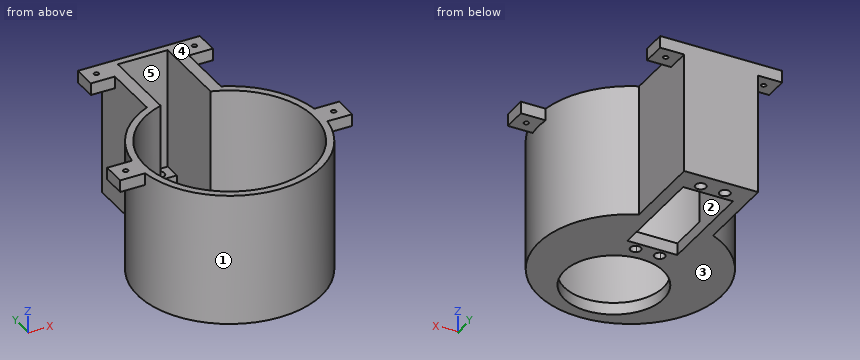
Autodesk Inventor part; units mm, degrees
ref_plane "YZ Plane" through (0, 0, 0) normal (1, 0, 0) x (0, 1, 0)
ref_plane "XZ Plane" through (0, 0, 0) normal (0, 1, 0) x (-1, 0, 0)
ref_plane "XY Plane" through (0, 0, 0) normal (0, 0, 1) x (1, 0, 0)
ref_plane "Work Plane1" through (0, 0, 0) normal (0, 0, 1) x (1, 0, 0)
sketch "Sketch1" plane through (0, 0, 0) normal (0, 0, 1) x (1, 0, 0)
  line L0 (10.3879, -20.2759) -> (10.3879, 20.2759)
  line L1 (-9.35, -21.3138) -> (9.35, -21.3138)
  line L2 (-10.3879, -21.3138) -> (10.3879, -21.3138)
  line L3 (10.3879, -21.3138) -> (10.3879, 21.3138)
  line L4 (10.3879, 21.3138) -> (-10.3879, 21.3138)
  line L5 (-10.3879, 21.3138) -> (-10.3879, -21.3138)
  line L6 (-10.3879, -21.3138) -> (10.3879, 21.3138) construction
  line L7 (10.3879, -21.3138) -> (-10.3879, 21.3138) construction
  line L8 (-15.3879, 31.3138) -> (15.3879, 31.3138)
  arc A0 (-6.25, 26.7) -> (-3.75, 26.7) centre (-5, 24.8896) ccw
  arc A1 (3.75, 26.7) -> (6.25, 26.7) centre (5, 24.8896) ccw
  arc A2 (-3.75, -26.7) -> (-6.25, -26.7) centre (-5, -24.8896) ccw
  arc A3 (6.25, -26.7) -> (3.75, -26.7) centre (5, -24.8896) ccw
  circle A4 centre (-5, 24.8896) radius 2.2
  circle A5 centre (5, 24.8896) radius 2.2
  circle A6 centre (-5, -24.8896) radius 2.2
  circle A7 centre (5, -24.8896) radius 2.2
  circle A8 centre (0, -50.7404) radius 20.6245
  arc A9 (-15.3879, -3.1452) -> (15.3879, -3.1452) centre (0, -38.1663) ccw
  arc A10 (0.0421, 0.0864) -> (-0.0421, 0.0864) centre (0, -38.1663) ccw
  line L9 (15.3879, 31.3138) -> (15.3879, -3.1452)
  line L10 (-15.3879, -3.1452) -> (-15.3879, 31.3138)
  point P0 (0, 0)
  dimension "d0" = 10.3879
  dimension "d5" = 10
extrude "Extrusion1" add sketch "Sketch1" along normal blind 5
sketch "Sketch2" plane through (0, 0, 5) normal (0, 0, 1) x (1, 0, 0)
  arc A0 (-15.3879, -3.1452) -> (15.3879, -3.1452) centre (0, -38.1663) ccw
  arc A1 (-15.3879, -3.1452) -> (15.3879, -3.1452) centre (0, -38.1663) ccw
  circle A2 centre (-5, -24.8896) radius 2.2
  circle A3 centre (5, -24.8896) radius 2.2
  circle A4 centre (0, -50.7404) radius 20.6245
  line L0 (-10.3879, -21.3138) -> (-10.3879, 21.3138)
  line L1 (10.3879, 21.3138) -> (10.3879, -21.3138)
  line L2 (10.3879, -21.3138) -> (-10.3879, -21.3138)
  line L3 (10.3879, -4.4789) -> (10.3879, -1.3511)
  line L4 (-10.3879, -1.3511) -> (-10.3879, -4.4789)
  line L5 (-15.3879, 31.3138) -> (15.3879, 31.3138)
  line L6 (15.3879, 31.3138) -> (15.3879, -3.1452)
  line L7 (-15.3879, -3.1452) -> (-15.3879, 31.3138)
  line L8 (10.3879, -4.4789) -> (10.3879, 21.3138)
  line L9 (-10.3879, 21.3138) -> (-10.3879, -4.4789)
  circle A5 centre (-5, 24.8896) radius 2.2
  circle A6 centre (5, 24.8896) radius 2.2
  circle A7 centre (0, -38.1663) radius 35.2526
  line L10 (10.3879, -4.4789) -> (10.3879, 28.3138)
  line L11 (10.3879, 28.3138) -> (-10.3879, 28.3138)
  line L12 (-10.3879, 28.3138) -> (-10.3879, -4.4789)
  point P0 (0, 0)
  dimension "d8" = 3
  dimension "d9" = 3
extrude "Extrusion2" add sketch "Sketch2" along normal blind 50 contours L7 L5 L6 A0
sketch "Sketch3" plane through (0, 0, 55) normal (0, 0, 1) x (1, 0, 0)
  line L0 (-15.3879, 31.3138) -> (-25.3879, 31.3138)
  line L1 (-25.3879, 31.3138) -> (-25.3879, 21.3138)
  line L2 (-25.3879, 21.3138) -> (-15.3879, 21.3138)
  line L3 (-15.3879, 31.3138) -> (-15.3879, -3.1452)
  line L4 (15.3879, 21.3138) -> (25.3879, 21.3138)
  line L5 (15.3879, -3.1452) -> (15.3879, 31.3138)
  line L6 (25.3879, 21.3138) -> (25.3879, 31.3138)
  line L7 (25.3879, 31.3138) -> (15.3879, 31.3138)
  arc A0 (-15.3879, -3.1452) -> (15.3879, -3.1452) centre (0, -38.1663) ccw
  line L8 (-25.3879, 31.3138) -> (-15.3879, 31.3138)
  line L9 (-15.3879, 31.3138) -> (-15.3879, 21.3138)
  line L10 (-15.3879, 21.3138) -> (-25.3879, 21.3138)
  line L11 (-25.3879, 21.3138) -> (-25.3879, 31.3138)
  line L12 (15.3879, 31.3138) -> (25.3879, 31.3138)
  line L13 (25.3879, 31.3138) -> (25.3879, 21.3138)
  line L14 (25.3879, 21.3138) -> (15.3879, 21.3138)
  line L15 (15.3879, 21.3138) -> (15.3879, 31.3138)
  circle A1 centre (-20.3879, 26.3138) radius 1
  circle A2 centre (20.3879, 26.3138) radius 1
  line L16 (-37.9245, -33.1663) -> (-48.2526, -33.1663)
  line L17 (-48.2526, -33.1663) -> (-48.2526, -43.1663)
  line L18 (-48.2526, -43.1663) -> (-37.9245, -43.1663)
  line L19 (-28.2526, -33.1663) -> (-48.2526, -43.1663) construction
  line L20 (-48.2526, -33.1663) -> (-28.2526, -43.1663) construction
  line L21 (-48.2526, -43.1663) -> (-38.2526, -43.1663)
  line L22 (-38.2526, -33.1663) -> (-48.2526, -33.1663)
  line L23 (-48.2526, -33.1663) -> (-48.2526, -43.1663)
  circle A3 centre (-43.2526, -38.1663) radius 1
  line L24 (48.2526, -33.1663) -> (37.9245, -33.1663)
  line L25 (37.9245, -43.1663) -> (48.2526, -43.1663)
  line L26 (48.2526, -43.1663) -> (48.2526, -33.1663)
  line L27 (48.2526, -33.1663) -> (28.2526, -43.1663) construction
  line L28 (28.2526, -33.1663) -> (48.2526, -43.1663) construction
  line L29 (48.2526, -43.1663) -> (38.2526, -43.1663)
  line L30 (38.2526, -33.1663) -> (48.2526, -33.1663)
  line L31 (48.2526, -33.1663) -> (48.2526, -43.1663)
  circle A4 centre (43.2526, -38.1663) radius 1
  circle A5 centre (0, -38.1663) radius 38.2526
  point P0 (0, 0)
  dimension "d14" = 20
  dimension "d15" = 10
  dimension "d16" = 2
  dimension "d18" = 10
  dimension "d19" = 2
extrude "Extrusion4" add sketch "Sketch3" against normal blind 5 contours L3 L2 L1 L0 | L5 L7 L6 L4 | A0 L18 L17 L16 | L24 L26 L25 A0
properties part number "Neck"
Input: part model. Units: mm. Frame: model coordinates. Face numbers are marked on the shaded views. A direction names the side the tool comes from. Round coordinates to 2 decimals unless told otherwise and drop trailing zeros. Order: outer loops, then holes, each group sorted by start corner. A loop starts at its lowest first (then second) coordinate and runs counter-clockwise, first axis right, second up.
1. Pin query (flat end, axial travel): P1, Ø2.5, axis at x = 20.39, y = 26.31, coming from the +Z side; P2, Ø1.5, axis at x = -44, z = 52.5, coming from the +Y side; P3, Ø3, axis at x = 43.25, y = -38.17, coming from the -Z side; P4, Ø25, axis at y = 10, z = 41, coming from the -X side. Return the tip coordinate at first contact, or that it passes through.
The answers:
P1: stops at z = 55
P2: stops at y = -33.17
P3: stops at z = 50
P4: stops at x = -15.39
2. Cut plane D-D, the plane z = 7. Output: boundary loops of the cut face in (x, y).
The answers:
outline: (-15.39, -3.15) arc R38.25 ccw (long way) to (15.39, -3.15) - (15.39, 31.31) - (-15.39, 31.31) - close; hole (-10.39, -4.48) arc R35.25 ccw (long way) to (10.39, -4.48) - (10.39, 28.31) - (-10.39, 28.31) - close
3. Cut plane B-B, the plane y = -61.5. Output: boundary loops of the cut face in (x, z), then the cut area to 3 significant figures.
The answers:
outline: (-30.31, 0) - (-17.6, 0) - (-17.6, 5) - (-26.43, 5) - (-26.43, 55) - (-30.31, 55) - close; (17.6, 0) - (30.31, 0) - (30.31, 55) - (26.43, 55) - (26.43, 5) - (17.6, 5) - close
area: 516 mm2
4. Cut plane A-A, the plane x = 0. Output: boundary loops of the cut face in (y, z).
The answers:
outline: (-76.42, 0) - (-71.36, 0) - (-71.36, 5) - (-73.42, 5) - (-73.42, 55) - (-76.42, 55) - close; (-30.12, 0) - (-21.31, 0) - (-21.31, 5) - (-30.12, 5) - close; (21.31, 0) - (31.31, 0) - (31.31, 55) - (28.31, 55) - (28.31, 5) - (21.31, 5) - close
5. Mould query, pull axis X, two halves, no side actions, for the marked faces 1, 2 and 3. Classes: released by +X, released by -X, zero draft, split by the parting line, or undercut.
The answers:
face 1: split by the parting line
face 2: undercut
face 3: zero draft
6. Set-up query: the marked faces 4 and 5. Return all of +Z, -Z, +X, -X, +Y, -Y with unobstructed straight access to the full face (end or side cutting, diameter ignored); none if empty.
The answers:
face 4: +Z, +X, -X, +Y, -Y
face 5: +Z
7. Material intervals for line 1 (X direction, y = 15, z = 46.5); line 2 (Y direction, x = 0, z = 21); line 3 (Y direction, x = 0, z = 1.75), sorted ascending.
The answers:
line 1: x = -15.39 to -10.39, 10.39 to 15.39
line 2: y = -76.42 to -73.42, 28.31 to 31.31
line 3: y = -76.42 to -71.36, -30.12 to -21.31, 21.31 to 31.31
8. Cut plane C-C, the plane x = -23.5. Output: boundary loops of the cut face in (y, z).
The answers:
outline: (-68.35, 0) - (-7.98, 0) - (-7.98, 55) - (-11.89, 55) - (-11.89, 5) - (-64.44, 5) - (-64.44, 55) - (-68.35, 55) - close; (21.31, 50) - (31.31, 50) - (31.31, 55) - (21.31, 55) - close
